For this review, use the dimensioned drawing (mm, ordinates from the lowest corner) and the shaded views. A direction names the side the tool comes from. Give positions to 0.01 mm unless a question says otherwise; leave off trailing zeros. Write each loop counter-clockwise with the first axis right and the second up, starting at its lowest first coordinate (ties: lowest second). Pieces come first, ordered by that corner, then holes. Notation, with made-up numbers: M 7,70 L 28,70 A9 cw 28,83 Z; hole C 26.5,-19 d6. An arc over 180 degrees is marked long. Write each question's results on one line, items separated by ' | '. Start each with the question number.
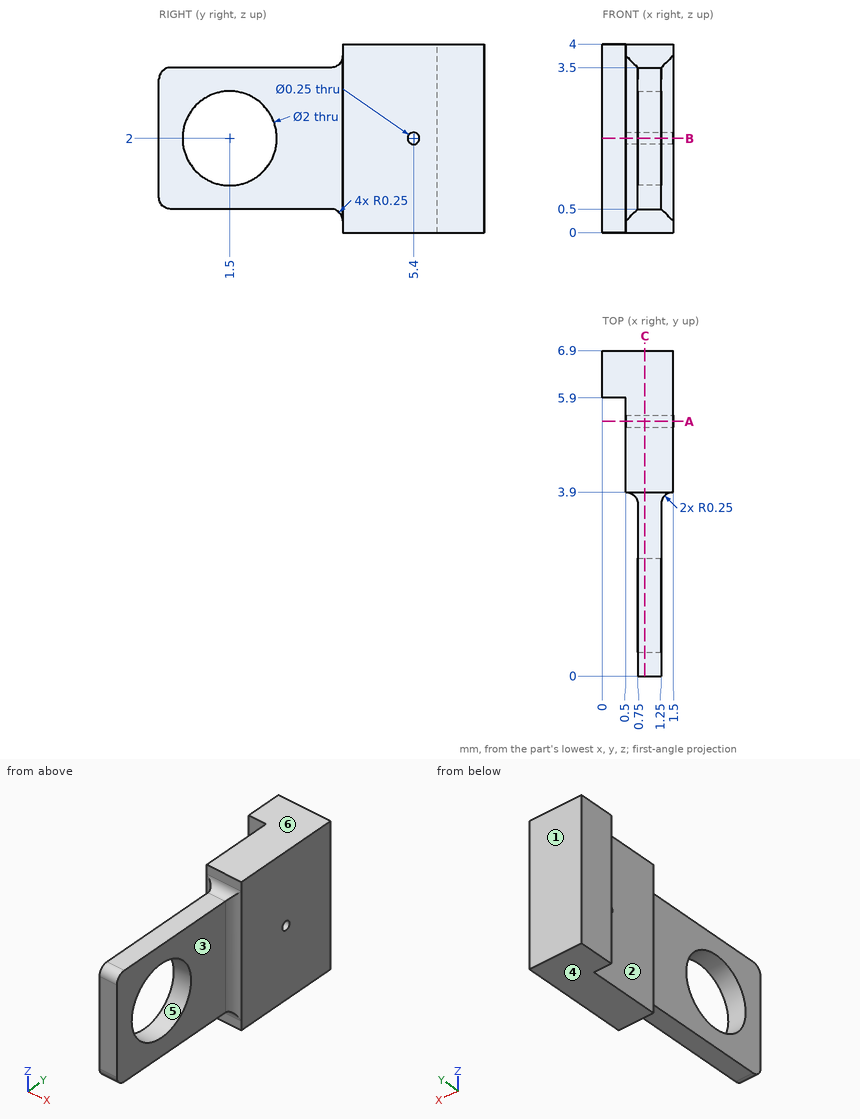
(1) Clearance check with flat-ended pins moving along their axes: P1, Ø0.6, axis at x = 1, y = 1, coming from the +Z side; P2, Ø1.8, axis at y = 1.5, z = 2, coming from the -X side; P3, Ø0.6, axis at x = 0.5, z = 2.5, coming from the -Y side; P4, Ø1.6, axis at y = 4.5, z = 1, coming from the -X side. State where each tip first meets the part, or that it passes through.
(2) Add section A-A (y = 5.4). State the section outline as (x, z) points (3 decimals), then the cut area to 3 significant figures.
(3) Add section C-C (x = 0.9). State the section outline as (y, z) points (3 decimals), then the cut area to 3 significant figures.
(4) Add section B-B (z = 2). Give the number of separate pieces and of enclosed holes in the cut face.
(5) Machinability: for the marked faces 1 and 2, which of the approach directions +Z, -Z, +X, -X, +Y, -Y give a long, thin tool a straight path to every point of the face, cutting with its end or side? Answer none if there is none.
(6) Draft analysis for pull direction Z (two halves, no side actions). For the marked faces 3, 4, 5 and 6, state which applies: pulls with the +Z half, pulls with the -Z half, needs draft (parallel to the pull), parting line crosses it, or undercut.
(7) Wall thickness on L1, parallel to Y at x = 1.15, z = 2 (3 decimals); L2, parallel to Z at x = 0.85, y = 5.4 (3 decimals); L3, parallel to X at y = 2.25, z = 3.2: over which ranges is each line inside the solid? List them lowest first.
Calculated:
1) P1: stops at z = 3.5 | P2: passes through | P3: stops at y = 0 | P4: stops at x = 0.5
2) outline: M 0.5,0 L 1.5,0 L 1.5,1.875 L 0.5,1.875 Z; M 0.5,2.125 L 1.5,2.125 L 1.5,4 L 0.5,4 Z | area: 3.75 mm²
3) outline: M 0,0.75 A0.25 ccw 0.25,0.5 L 3.65,0.5 A0.25 cw 3.9,0.25 L 3.9,0 L 6.9,0 L 6.9,4 L 3.9,4 L 3.9,3.75 A0.25 cw 3.65,3.5 L 0.25,3.5 A0.25 ccw 0,3.25 Z; hole C 1.5,2 d2; hole C 5.4,2 d0.25 | area: 20.5 mm²
4) separate pieces: 3 | enclosed holes: 0
5) face 1: +Z, -Z, +X, -X, +Y | face 2: +Z, -Z, -X, -Y
6) face 3: needs draft | face 4: pulls with the -Z half | face 5: undercut | face 6: pulls with the +Z half
7) L1: y = 0 to 0.5, 2.5 to 5.275, 5.525 to 6.9 | L2: z = 0 to 1.875, 2.125 to 4 | L3: x = 0.75 to 1.25
